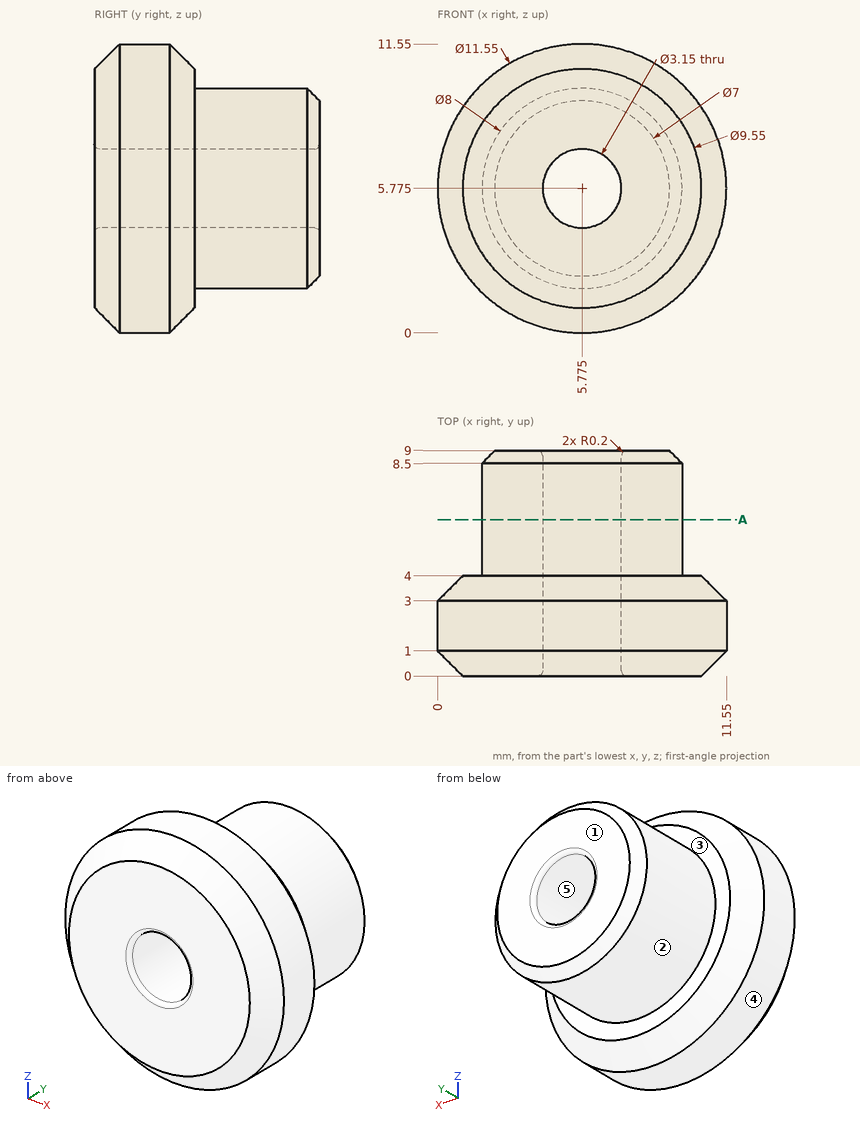
The drawing under review shows one solid part. Ordinate dimensions are in mm from its lowest x, y, z. A direction names the side the tool comes from. Coordinates: 2 decimals unless noted, no trailing zeros. Loops run counter-clockwise (first coordinate to the right, second up) from the corner with the lowest first, then second, coordinate; pieces in that order, holes last. Notation, with made-up numbers: (32, 8.25) - (45, 8.25) arc R22 ccw to (45, 42.25) - close; hole circle Ø11 at (25.5, 39.25). An arc over 180 degrees is marked (long way). Return JSON: item names as keys, results as strings.
Item 1: Insertion check: pin 1 (2 mm diameter, centred on y = 6.5, z = 6, fed in from -X) (3 decimals); pin 2 (3 mm diameter, centred on x = 5.775, z = 5.775, fed in from -Y); pin 3 (4 mm diameter, centred on x = 2, y = 5.5, fed in from +Z); pin 4 (3 mm diameter, centred on y = 1.5, z = 3, fed in from -X). Each pin has a flat end and moves straight along its axis. Give the tip position at first contact, or say it passes through.
Determined:
{"pin 1": "stops at x = 1.775", "pin 2": "passes through", "pin 3": "stops at z = 9.94", "pin 4": "stops at x = 0.14"}
Item 2: Take a section at A-A (y = 6.25). Give the boundary of the cut face in (x, z) (3 decimals).
Determined:
{"outline": "circle Ø8 at (5.775, 5.775); hole circle Ø3.15 at (5.775, 5.775)"}
Item 3: Mouldability with a two-part tool opening along X and no side actions: class the marked faces 3, 4 and 5 as pulls with the +X half, pulls with the -X half, needs draft (parallel to the pull), parting line crosses it, or undercut.
Determined:
{"face 3": "needs draft", "face 4": "parting line crosses it", "face 5": "undercut"}
Item 4: For the marked faces 1 and 2, list the 3-axis set-ups (+Z, -Z, +X, -X, +Y, -Y) from which the entire face can be reached by the end or side of a thin tool; tool diameter is ignored.
Determined:
{"face 1": "+Z, -Z, +X, -X, +Y", "face 2": "+Y"}
Item 5: For line 1 (X direction, y = 7.75, z = 5.75); line 2 (X direction, y = 5, z = 4.5); line 3 (Y direction, x = 2, z = 8), list the stretches that pass through material, from the lowest coordinate up.
Determined:
{"line 1": "x = 1.78 to 4.2, 7.35 to 9.77", "line 2": "x = 1.98 to 4.85, 6.7 to 9.57", "line 3": "y = 0 to 4"}
